Input: part model. Units: mm. Frame: model coordinates. Face numbers are marked on the shaded views. Coordinates: 2 decimals unless noted, no trailing zeros. Loops run counter-clockwise (first coordinate to the right, second up) from the corner with the lowest first, then second, coordinate; pieces in that order, holes last. Notation, with made-up numbers: (1, -15.5) -> (60, -15.5) arc R11 ccw to (60, 2.5) -> close; hole circle Ø10 at (64, 18). An arc over 180 degrees is marked (long way). Answer as a JSON object with one key per item and string values.
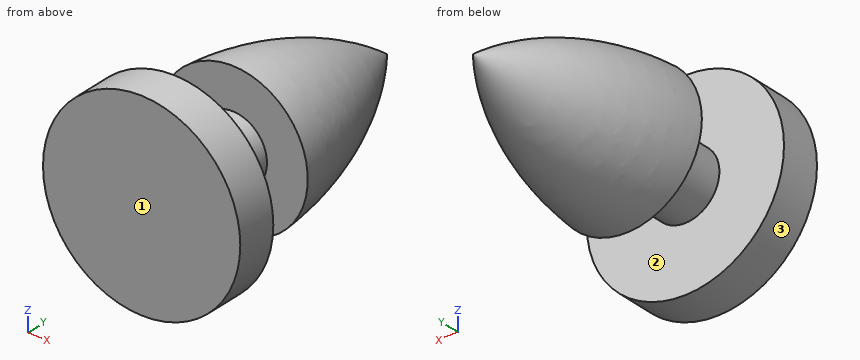
Autodesk Inventor part; units mm, degrees
ref_plane "Work Plane1" through (0, 8.3, 0) normal (0, 1, 0) x (1, 0, 0)
ref_plane "YZ Plane" through (0, 0, 0) normal (1, 0, 0) x (0, 1, 0)
ref_plane "XZ Plane" through (0, 0, 0) normal (0, 1, 0) x (-1, 0, 0)
sketch "Sketch1" plane through (0, 0, 0) normal (0, 1, 0) x (-1, 0, 0)
  circle A0 centre (0, 0) radius 7.25
  dimension "d0" = 14.5
extrude "Extrusion1" add sketch "Sketch1" along normal blind 3
sketch "Sketch2" plane through (0, 3, 0) normal (0, 1, 0) x (1, 0, 0)
  circle A0 centre (0, 0) radius 2.5
  dimension "d3" = 5
extrude "Extrusion2" add sketch "Sketch2" along normal blind 14.7
ref_plane "Work Plane1" through (0, 8.3, 0) normal (0, 1, 0) x (1, 0, 0)
sketch "Sketch4" plane through (0, 0, 0) normal (0, 0, 1) x (1, 0, 0)
  line L0 (0, 0) -> (0, 8.2998)
  line L1 (0, 8.2998) -> (-5.5, 8.2998)
  line L2 (2.5, 17.7) -> (-2.5, 17.7)
  line L3 (0, 22.2998) -> (0, 8.2998)
  arc A0 (0, 22.2998) -> (-5.5, 8.2998) centre (20.0135, 6.357) ccw
  line L4 (0, 22.2998) -> (0, 30.2311)
  dimension "d8" = 5.5
  dimension "d9" = 14
revolve "Revolution1" add sketch "Sketch4" angle 360 about axis through (0, 22.2998, 0) along (0, 1, 0)
properties part number "MotorMountingHub"
1. Line query: line 1 along Y through (x, z) = (0.25, -3.25); line 2 along Y through (x, z) = (6.25, 2.25); line 3 along Y through (x, z) = (2, 3.25). Output: solid intervals per line, ascending.
Reply:
{"line 1": "y = 0 to 3, 8.3 to 16.99", "line 2": "y = 0 to 3", "line 3": "y = 0 to 3, 8.3 to 15.68"}
2. Section query A-A (y = 2). Return loops of the section in (x, z), plus the area to 3 significant figures.
Reply:
{"outline": "circle Ø14.5 at (0, 0)", "area": "165 mm2"}
3. Mould query, pull axis Y, two halves, no side actions, for the marked faces 1, 2 and 3. Classes: pulls with the +Y half, pulls with the -Y half, needs draft (parallel to the pull), parting line crosses it, or undercut.
Reply:
{"face 1": "pulls with the -Y half", "face 2": "undercut", "face 3": "needs draft"}
4. Pin query (flat end, axial travel): P1, Ø3, axis at x = -2.5, y = 7, coming from the -Z side; P2, Ø4.5, axis at x = 1.5, z = -3, coming from the +Y side; P3, Ø3, axis at y = 6.5, z = -2, coming from the +X side. Return the tip coordinate at first contact, or that it passes through.
Reply:
{"P1": "stops at z = -5.21", "P2": "stops at y = 20.81", "P3": "stops at x = 2.45"}
